Autodesk Inventor part; units mm, degrees
ref_plane "YZ Plane" through (0, 0, 0) normal (1, 0, 0) x (0, 1, 0)
ref_plane "XZ Plane" through (0, 0, 0) normal (0, 1, 0) x (-1, 0, 0)
ref_plane "XY Plane" through (0, 0, 0) normal (0, 0, 1) x (1, 0, 0)
sketch "Sketch1" plane through (0, 0, 0) normal (0, 1, 0) x (-1, 0, 0)
  line L0 (0, 0) -> (10, 0)
  line L1 (10, 0) -> (10, -125)
  line L2 (10, -125) -> (0, -125)
  line L3 (0, -125) -> (0, 0)
  line L4 (27.7651, -45) -> (-20.7182, -45) construction
  circle A0 centre (5, -100) radius 2.5
  circle A1 centre (5, -75) radius 2.5
  point P0 (5, -13.5)
  dimension "d0" = 125
  dimension "d1" = 10
  dimension "d2" = 25
  dimension "d3" = 25
  dimension "d4" = 80
  dimension "d7" = 5
  dimension "d9" = 5
  dimension "d11" = 31.5
extrude "Extrusion1" add sketch "Sketch1" along normal blind 1
fillet "Fillet1" radius 1 1 edges at (0, 0.5, -125)
fillet "Fillet2" radius 1 3 edges at (0, 0.5, 0) (-10, 0.5, 0) (-10, 0.5, -125)
properties part number "ConnectorStrip"
Could you check a few things on this model? Use its own coordinates, in mm. Round coordinates to 2 decimals unless told otherwise and drop trailing zeros. Write each loop counter-clockwise with the first axis right and the second up, starting at its lowest first coordinate (ties: lowest second). Pieces come first, ordered by that corner, then holes. Notation, with made-up numbers: (43, 61.5) -> (72, 61.5) arc R29 ccw to (72, 96.5) -> close; hole circle Ø3 at (28, -13.5). An arc over 180 degrees is marked (long way). Use a Markdown table: item, result.
1. We'd pull the mould along Z, two halves only. Please class faces 1 (the face through (-4.67, 0.49, -102.48)), 2 (the face through (-5, 1, -62)): +Z half, -Z half, draft (parallel to the pull), parting line (faces both ways), or undercut.
Answer key:
| item | result |
|---|---|
| face 1 | undercut |
| face 2 | draft |
2. If we section it at B-B (x = -5): List the corners of the cut face in (y, z) for me.
Answer key:
| item | result |
|---|---|
| outline | (0, -125) -> (1, -125) -> (1, -102.5) -> (0, -102.5) -> close; (0, -97.5) -> (1, -97.5) -> (1, -77.5) -> (0, -77.5) -> close; (0, -72.5) -> (1, -72.5) -> (1, 0) -> (0, 0) -> close |
3. For pin 1 Ø4 at (x, z) = (-6, -69.5) entering from -Y, with a flat end and sliding along its axis, tell me the tip position at first contact or that it passes through.
Answer key:
| item | result |
|---|---|
| pin 1 | stops at y = 0 |
4. Please list where these lines run through material, in increasing order: probe 1 along Z at (x, y) = (-5, 0.55); probe 2 along Z at (x, y) = (-6.75, 0.75); probe 3 along Z at (x, y) = (-0.5, 0.4).
Answer key:
| item | result |
|---|---|
| probe 1 | z = -125 to -102.5, -97.5 to -77.5, -72.5 to 0 |
| probe 2 | z = -125 to -101.79, -98.21 to -76.79, -73.21 to 0 |
| probe 3 | z = -124.87 to -0.13 |
5. If we section it at A-A (z = -100): List the corners of the cut face in (x, y) for me.
Answer key:
| item | result |
|---|---|
| outline | (-10, 0) -> (-7.5, 0) -> (-7.5, 1) -> (-10, 1) -> close; (-2.5, 0) -> (0, 0) -> (0, 1) -> (-2.5, 1) -> close |
6. If we section it at C-C (y = 0.6): List the corners of the cut face in (x, z) for me, then the cut area to 3 significant figures.
Answer key:
| item | result |
|---|---|
| outline | (-10, -124) arc R1 ccw to (-9, -125) -> (-1, -125) arc R1 ccw to (0, -124) -> (0, -1) arc R1 ccw to (-1, 0) -> (-9, 0) arc R1 ccw to (-10, -1) -> close; hole circle Ø5 at (-5, -100); hole circle Ø5 at (-5, -75) |
| area | 1,210 mm^2 |
